from build123d import *

# Parameters (mm, degrees)
SKETCH1_W           = 19.05
SKETCH1_H           = 95.25
BOSS_EXTRUDE2_DEPTH = 2.54


with BuildPart() as part:
    # Sketch1 → Boss-Extrude2 (new body)
    with BuildSketch(Plane.XY):
        with BuildLine():
            Line((-362.508916396, 81.370262461), (-362.508916396, 64.860262461))
            ThreePointArc((-362.508916396, 64.860262461), (-359.968916396, 62.320262461), (-362.508916396, 59.780262461))
            Line((-362.508916396, 59.780262461), (-362.508916396, -11.339737539))
            ThreePointArc((-362.508916396, -11.339737539), (-359.968916396, -13.879737539), (-362.508916396, -16.419737539))
            Line((-362.508916396, -16.419737539), (-362.508916396, -20.229737539))
            Line((-362.508916396, -20.229737539), (81.991083604, -20.229737539))
            Line((81.991083604, -20.229737539), (81.991083604, -16.419737539))
            ThreePointArc((81.991083604, -16.419737539), (79.451083604, -13.879737539), (81.991083604, -11.339737539))
            Line((81.991083604, -11.339737539), (81.991083604, 59.780262461))
            ThreePointArc((81.991083604, 59.780262461), (79.451083604, 62.320262461), (81.991083604, 64.860262461))
            Line((81.991083604, 64.860262461), (81.991083604, 81.370262461))
            Line((81.991083604, 81.370262461), (-362.508916396, 81.370262461))
        make_face()
        with Locations((-64.058916396, 30.570262461)):
            Rectangle(SKETCH1_W, SKETCH1_H, mode=Mode.SUBTRACT)
        Polygon((-316.407916396, 11.451682461), (-316.407916396, 36.851682461), (-292.658916396, 36.851682461), (-268.909916396, 36.851682461), (-268.909916396, 11.451682461), (-292.658916396, 11.451682461), align=None, mode=Mode.SUBTRACT)
        Polygon((-164.007916396, 11.451682461), (-164.007916396, 36.851682461), (-140.258916396, 36.851682461), (-116.509916396, 36.851682461), (-116.509916396, 11.451682461), (-140.258916396, 11.451682461), align=None, mode=Mode.SUBTRACT)
        with Locations((-216.458916396, 30.570262461)):
            Rectangle(SKETCH1_W, SKETCH1_H, mode=Mode.SUBTRACT)
        Polygon((-11.607916396, 11.451682461), (-11.607916396, 36.851682461), (12.141083604, 36.851682461), (35.890083604, 36.851682461), (35.890083604, 11.451682461), (12.141083604, 11.451682461), align=None, mode=Mode.SUBTRACT)
    extrude(amount=BOSS_EXTRUDE2_DEPTH)


solid = part.part
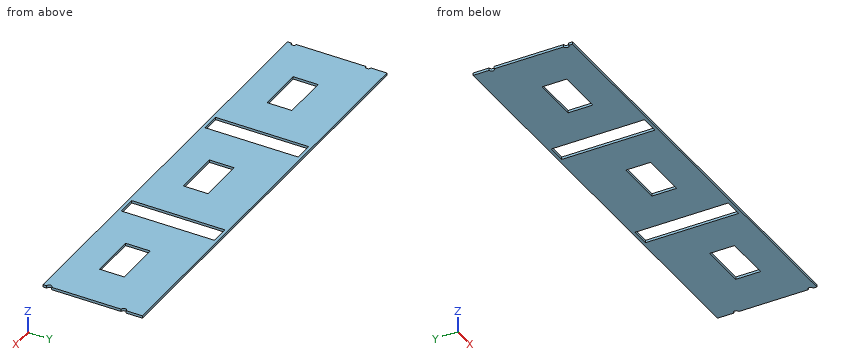
Model file for the job. Use its own axes, mm. Coordinates: 2 decimals unless noted, no trailing zeros. Order: outer loops, then holes, each group sorted by start corner. A loop starts at its lowest first (then second) coordinate and runs counter-clockwise, first axis right, second up. Notation, with made-up numbers: (27, 9.5) -> (60, 9.5) arc R10 cw to (60, 19.5) -> close; hole circle Ø4 at (28, 14.5). An arc over 180 degrees is marked (long way). Return JSON: item names as keys, results as strings. Group by question number.
Item 1: Saw through at D-D on y = 24.5. Write the cut outline in (x, z).
Item 2: Saw through at C-C on y = 45.5. Write the cut outline in (x, z).
Item 3: Saw through at B-B on z = 0.5. State how many separate pieces and enclosed holes the cut face has, then the cut area to 3 significant figures.
Item 4: Saw through at A-A on x = -5. Write the cut outline in (y, z).
Item 5: Wall check: line 1 along X through (y, z) = (48, 0.85); line 2 along X through (y, z) = (25, 0.75); line 3 along Y through (x, z) = (-284.5, 0.8). Give the ranges that are in metal, low to high. Write a range as [from, to].
Values found:
{
 "1": {"outline": "(-362.51, 0) -> (-316.41, 0) -> (-316.41, 2.54) -> (-362.51, 2.54) -> close; (-268.91, 0) -> (-225.98, 0) -> (-225.98, 2.54) -> (-268.91, 2.54) -> close; (-206.93, 0) -> (-164.01, 0) -> (-164.01, 2.54) -> (-206.93, 2.54) -> close; (-116.51, 0) -> (-73.58, 0) -> (-73.58, 2.54) -> (-116.51, 2.54) -> close; (-54.53, 0) -> (-11.61, 0) -> (-11.61, 2.54) -> (-54.53, 2.54) -> close; (35.89, 0) -> (81.99, 0) -> (81.99, 2.54) -> (35.89, 2.54) -> close"},
 "2": {"outline": "(-362.51, 0) -> (-225.98, 0) -> (-225.98, 2.54) -> (-362.51, 2.54) -> close; (-206.93, 0) -> (-73.58, 0) -> (-73.58, 2.54) -> (-206.93, 2.54) -> close; (-54.53, 0) -> (81.99, 0) -> (81.99, 2.54) -> (-54.53, 2.54) -> close"},
 "3": {"separate pieces": "1", "enclosed holes": "5", "area": "37,900 mm2"},
 "4": {"outline": "(-20.23, 0) -> (11.45, 0) -> (11.45, 2.54) -> (-20.23, 2.54) -> close; (36.85, 0) -> (81.37, 0) -> (81.37, 2.54) -> (36.85, 2.54) -> close"},
 "5": {"line 1": "x = [-362.51, -225.98], [-206.93, -73.58], [-54.53, 81.99]", "line 2": "x = [-362.51, -316.41], [-268.91, -225.98], [-206.93, -164.01], [-116.51, -73.58], [-54.53, -11.61], [35.89, 81.99]", "line 3": "y = [-20.23, 11.45], [36.85, 81.37]"}
}
